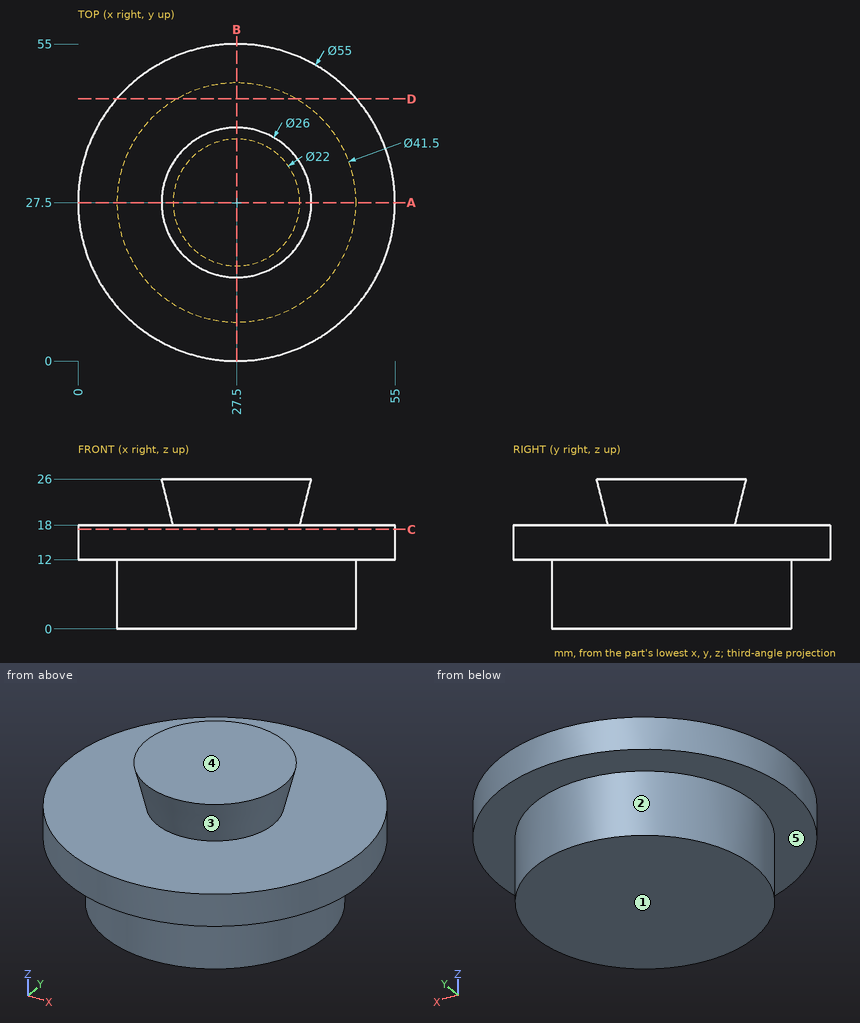
The drawing under review shows one solid part. Ordinate dimensions are in mm from its lowest x, y, z. A direction names the side the tool comes from. Coordinates: 2 decimals unless noted, no trailing zeros. Write each loop counter-clockwise with the first axis right and the second up, starting at its lowest first coordinate (ties: lowest second). Pieces come first, ordered by that corner, then holes.
1) Add section D-D (y = 45.5). Write out the cut boundary in (x, z), plus the area to 3 significant figures.
2) To check wall thickness, follow L1, parallel to Z at x = 19.5, y = 42.5; L2, parallel to Z at x = 42.5, y = 10; L3, parallel to X at y = 33, z = 19. State the ranges of each line that lie inside material, in increasing order.
3) Mouldability with a two-part tool opening along Z and no side actions: class the marked faces 3, 4 and 5 as +Z half, -Z half, draft (parallel to the pull), parting line (faces both ways), or undercut.
4) Machinability: for the marked faces 1 and 2, which of the approach directions +Z, -Z, +X, -X, +Y, -Y give a long, thin tool a straight path to every point of the face, cutting with its end or side? Answer none if there is none.
5) Insertion check: pin 1 (8 mm diameter, centred on x = 36.5, z = 13.5, fed in from -Y); pin 2 (6 mm diameter, centred on y = 5.5, z = 5.5, fed in from -X); pin 3 (2 mm diameter, centred on y = 16.5, z = 4.5, fed in from +X). Each pin has a flat end and moves straight along its axis. Give the tip position at first contact, or say it passes through.
6) Add section A-A (y = 27.5). Write out the cut boundary in (x, z), plus the area to 3 significant figures.
7) Add section C-C (z = 17.25). Write out the cut boundary in (x, y), plus the area to 3 significant figures.
Check result:
1. outline: (6.71, 12) - (17.18, 12) - (17.18, 0) - (37.82, 0) - (37.82, 12) - (48.29, 12) - (48.29, 18) - (6.71, 18) - close
1. area: 497 mm2
2. L1: z = 0 to 18
2. L2: z = 12 to 18
2. L3: x = 17.69 to 37.31
3. face 3: undercut
3. face 4: +Z half
3. face 5: -Z half
4. face 1: -Z, +X, -X, +Y, -Y
4. face 2: -Z
5. pin 1: stops at y = 0.46
5. pin 2: stops at x = 19.16
5. pin 3: stops at x = 45.68
6. outline: (0, 12) - (6.75, 12) - (6.75, 0) - (48.25, 0) - (48.25, 12) - (55, 12) - (55, 18) - (38.5, 18) - (40.5, 26) - (14.5, 26) - (16.5, 18) - (0, 18) - close
6. area: 1,020 mm2
7. outline: circle Ø55 at (27.5, 27.5)
7. area: 2,380 mm2
